Part model, mm, in its own coordinate system. A direction names the side the tool comes from. Coordinates: 2 decimals unless noted, no trailing zeros. Write each loop counter-clockwise with the first axis right and the second up, starting at its lowest first coordinate (ties: lowest second). Pieces come first, ordered by that corner, then holes. Notation, with made-up numbers: (-37.75, -2.75) -> (-1.75, -2.75) arc R34 cw to (-1.75, 31.25) -> close; hole circle Ø6 at (0.25, 1.5). An arc over 180 degrees is marked (long way). Write item = value, one per line.
from build123d import *
from OCP.BRepFilletAPI import BRepFilletAPI_MakeFillet

# Parameters (mm, degrees)
BOSS_EXTRUDE1_DEPTH                                 = 20
CBORE_FOR_M4_HEX_SOCKET_HEAD_CAP_SCREW1_D           = 4.5
CBORE_FOR_M4_HEX_SOCKET_HEAD_CAP_SCREW1_DEPTH       = 10
CBORE_FOR_M4_HEX_SOCKET_HEAD_CAP_SCREW1_CBORE_D     = 8
CBORE_FOR_M4_HEX_SOCKET_HEAD_CAP_SCREW1_CBORE_DEPTH = 4.4
BOSS_EXTRUDE3_DEPTH                                 = 7.8
CUT_EXTRUDE1_DEPTH                                  = 2.4
FILLET3_R                                           = 0.5
CUT_SWEEP1_START                                    = -2.5
CUT_SWEEP1_DEPTH                                    = 5
CUT_EXTRUDE2_REACH                                  = 67.401
SKETCH14_R                                          = 4
FILLET4_R1                                          = 1
FILLET4_R2                                          = 5


# Read off the part's stored shape, not the designer's step: Cut-Sweep1
with BuildPart() as part:
    # Sketch1 → Boss-Extrude1 (new, symmetric)
    with BuildSketch(Plane.XY):
        Polygon((-12.5, 10), (7.5, 10), (7.5, 50), (-7.5, 50), (-7.5, 53), (12.5, 53), (12.5, 0), (-12.5, 0), align=None)
    extrude(amount=BOSS_EXTRUDE1_DEPTH, both=True)

    # CBORE for M4 Hex Socket Head Cap Screw1
    with Locations(Plane(origin=(0, 10, 0), x_dir=(1, 0, 0), z_dir=(0, 1, 0))):
        with Locations((0, -13)):
            CounterBoreHole(CBORE_FOR_M4_HEX_SOCKET_HEAD_CAP_SCREW1_D / 2, CBORE_FOR_M4_HEX_SOCKET_HEAD_CAP_SCREW1_CBORE_D / 2, CBORE_FOR_M4_HEX_SOCKET_HEAD_CAP_SCREW1_CBORE_DEPTH, depth=CBORE_FOR_M4_HEX_SOCKET_HEAD_CAP_SCREW1_DEPTH)

    # Sketch5 → Boss-Extrude3 (add)
    with BuildSketch(Plane(origin=(0, 0, -20), x_dir=(-1, 0, 0), z_dir=(0, 0, -1))):
        Polygon((-5, -8), (5, -8), (8.25, -4.4), (8.25, -2.4), (3.9, -2.4), (3.9, 0), (-3.9, 0), (-3.9, -2.4), (-8.25, -2.4), (-8.25, -4.4), align=None)
    extrude(amount=-BOSS_EXTRUDE3_DEPTH)

    # Sketch6 → Cut-Extrude1 (cut)
    with BuildSketch(Plane(origin=(0, -2.4, 0), x_dir=(1, 0, 0), z_dir=(0, 1, 0))):
        with BuildLine():
            ThreePointArc((-3.9, 16.1), (-2.757716447, 18.857716447), (0, 20))
            Line((0, 20), (-3.9, 20))
            Line((-3.9, 20), (-3.9, 16.1))
        make_face()
        with BuildLine():
            Line((3.9, 12.2), (3.9, 16.1))
            ThreePointArc((3.9, 16.1), (2.757716447, 13.342283553), (0, 12.2))
            Line((0, 12.2), (3.9, 12.2))
        make_face()
    extrude(amount=CUT_EXTRUDE1_DEPTH, mode=Mode.SUBTRACT)

    # Fillet3
    fillet3_edges = [part.edges().sort_by_distance(p)[0] for p in [
        (3.9, 0, -18.05),
        (2.757716447, 0, -13.342283553),
        (-1.95, 0, -12.2),
    ]]
    fillet(fillet3_edges, radius=FILLET3_R)
    fillet3_2_edges = [part.edges().sort_by_distance(p)[0] for p in [
        (-3.9, 0, -14.15),
        (-2.757716447, 0, -18.857716447),
    ]]
    fillet(fillet3_2_edges, radius=FILLET3_R)
    fillet3_3_edges = [part.edges().sort_by_distance(p)[0] for p in [
        (-8.25, -2.4, -16.1),
    ]]
    fillet(fillet3_3_edges, radius=FILLET3_R)
    fillet3_4_edges = [part.edges().sort_by_distance(p)[0] for p in [
        (-8.25, -4.4, -16.1),
    ]]
    fillet(fillet3_4_edges, radius=FILLET3_R)
    fillet3_5_edges = [part.edges().sort_by_distance(p)[0] for p in [
        (-5, -8, -16.1),
    ]]
    fillet(fillet3_5_edges, radius=FILLET3_R)
    fillet3_6_edges = [part.edges().sort_by_distance(p)[0] for p in [
        (5, -8, -16.1),
    ]]
    fillet(fillet3_6_edges, radius=FILLET3_R)
    fillet3_7_edges = [part.edges().sort_by_distance(p)[0] for p in [
        (8.25, -4.4, -16.1),
    ]]
    fillet(fillet3_7_edges, radius=FILLET3_R)
    fillet3_8_edges = [part.edges().sort_by_distance(p)[0] for p in [
        (8.25, -2.4, -16.1),
    ]]
    fillet(fillet3_8_edges, radius=FILLET3_R)

    # Cut-Sweep1 outline → Cut-Sweep1 (cut)
    with BuildSketch(Plane.XY.offset(CUT_SWEEP1_START)):
        with BuildLine():
            Line((12.500000017, 40.338970285), (12.5, 45.105483834))
            add(Edge.make_bspline(
                [(12.5, 45.105483834), (12.059714128, 45.789978249), (11.581411154, 46.38791258), (10.025035585, 47.892146935), (8.787180136, 48.5), (7.5, 48.5)],
                knots=[0.656472281, 0.656472281, 0.656472281, 0.656472281, 0.6875, 0.6875, 0.75, 0.75, 0.75, 0.75], degree=3))
            Line((7.5, 48.5), (7.5, 46.5))
            add(Edge.make_bspline(
                [(12.500000017, 40.338970285), (12.309154865, 40.920252732), (12.103143429, 41.469478304), (11.227294674, 43.513125401), (10.449149583, 44.700789342), (8.901182872, 46.196896563), (8.176315005, 46.5), (7.5, 46.5)],
                knots=[0.604163443, 0.604163443, 0.604163443, 0.604163443, 0.625, 0.625, 0.6875, 0.6875, 0.75, 0.75, 0.75, 0.75], degree=3))
        make_face()
        with BuildLine():
            Line((12.5, 14.894516166), (12.500000017, 19.661029715))
            add(Edge.make_bspline(
                [(7.5, 13.5), (8.176315005, 13.5), (8.901182872, 13.803103437), (10.449149583, 15.299210658), (11.227294674, 16.486874599), (12.103143429, 18.530521696), (12.309154865, 19.079747268), (12.500000017, 19.661029715)],
                knots=[0.25, 0.25, 0.25, 0.25, 0.3125, 0.3125, 0.375, 0.375, 0.395836557, 0.395836557, 0.395836557, 0.395836557], degree=3))
            Line((7.5, 13.5), (7.5, 11.5))
            add(Edge.make_bspline(
                [(7.5, 11.5), (8.787180136, 11.5), (10.025035585, 12.107853065), (11.581411154, 13.61208742), (12.059714128, 14.210021751), (12.5, 14.894516166)],
                knots=[0.25, 0.25, 0.25, 0.25, 0.3125, 0.3125, 0.343527719, 0.343527719, 0.343527719, 0.343527719], degree=3))
        make_face()
    extrude(amount=CUT_SWEEP1_DEPTH, mode=Mode.SUBTRACT)

    # Sketch14 → Cut-Extrude2 (cut, up to next)
    with BuildSketch(Plane(origin=(0, 53, 0), x_dir=(1, 0, 0), z_dir=(0, 1, 0)), mode=Mode.PRIVATE) as cut_extrude2_sk1:
        Polygon((-7.5, -20), (5.5, -20), (5.5, -9), (0, -9), (-7.5, -9), align=None)
        with BuildLine():
            ThreePointArc((4, -13), (-2.828427125, -15.828427125), (0, -9))
            ThreePointArc((0, -9), (2.828427125, -10.171572875), (4, -13))
        make_face(mode=Mode.SUBTRACT)
    cut_extrude2_tool1 = extrude(cut_extrude2_sk1.sketch, amount=-CUT_EXTRUDE2_REACH, mode=Mode.PRIVATE) & part.part
    # Sketch14 → Cut-Extrude2 (cut, up to next)
    with BuildSketch(Plane(origin=(0, 53, 0), x_dir=(1, 0, 0), z_dir=(0, 1, 0)), mode=Mode.PRIVATE) as cut_extrude2_sk2:
        with Locations(Location((0, -13, 0), (0, 0, 270))):
            Circle(SKETCH14_R)
    cut_extrude2_tool2 = extrude(cut_extrude2_sk2.sketch, amount=-CUT_EXTRUDE2_REACH, mode=Mode.PRIVATE) & part.part
    add(cut_extrude2_tool1.solids().sort_by_distance((-1, 53, 19.829706))[0], mode=Mode.SUBTRACT)
    add(cut_extrude2_tool2.solids().sort_by_distance((0, 53, 13))[0], mode=Mode.SUBTRACT)

    # Fillet4: one fillet with a radius per group of edges: ONE call of the kernel's fillet builder (fillet() takes one radius for all edges)
    fillet4_edges_1 = [part.edges().sort_by_distance(p)[0] for p in [
        (-12.5, 10, 0),
        (7.5, 10, 0),
        (7.5, 50, 0),
        (12.5, 53, 0),
        (12.5, 0, 0),
        (-12.5, 0, 0),
        (-7.5, 51.5, 9),
        (-7.5, 51.5, -20),
    ]]
    fillet4_edges_2 = [part.edges().sort_by_distance(p)[0] for p in [
        (5.5, 51.5, 9),
    ]]
    fillet4 = BRepFilletAPI_MakeFillet(part.part.solid().wrapped)
    for e in fillet4_edges_1:
        fillet4.Add(FILLET4_R1, e.wrapped)
    for e in fillet4_edges_2:
        fillet4.Add(FILLET4_R2, e.wrapped)
    add(Compound.cast(fillet4.Shape()), mode=Mode.REPLACE)


solid = part.part
Q1. Saw through at B-B on z = 13. Give the cut face in (x, y), and give its area (3 significant figures).
Model answer:
outline = (-12.5, 1) arc R1 ccw to (-11.5, 0) -> (-2.25, 0) -> (-2.25, 5.6) -> (-4, 5.6) -> (-4, 10) -> (-11.5, 10) arc R1 ccw to (-12.5, 9) -> close; (2.25, 0) -> (11.5, 0) arc R1 ccw to (12.5, 1) -> (12.5, 52) arc R1 ccw to (11.5, 53) -> (5.4, 53) -> (5.4, 50) -> (6.5, 50) arc R1 cw to (7.5, 49) -> (7.5, 11) arc R1 cw to (6.5, 10) -> (4, 10) -> (4, 5.6) -> (2.25, 5.6) -> close
area = 410 mm²
Q2. Probe line 1 (Z direction, x = 0, y = 3.95); line 2 (X direction, y = 2.3, z = 13); line 3 (Y direction, x = 8.25, z = 0). List the from-to ranges inside material, lowest first. Write a range as from..to.
Model answer:
line_1 = -20..10.75, 15.25..20
line_2 = -12.5..-2.25, 2.25..12.5
line_3 = 0..11.57, 13.62..46.38, 48.43..53
Q3. Pin check, flat tips, straight feed: pin 1 (11.5 mm diameter, centred on x = -1.5, z = 0, fed in from -Y); pin 2 (19 mm diameter, centred on y = 21, z = -3.5, fed in from -X); pin 3 (3.5 mm diameter, centred on x = -4, y = 51.5, fed in from +Z). Stop position of each tip, or through.
Model answer:
pin_1 = 0
pin_2 = 7.5
pin_3 = 9
Q4. Mould opens along X. For faces 5 (the face through (0, 50, -4)), 6 (the face through (10, 46, -2.5)), 7 (the face through (10, 46, 2.5)), 8 (the face through (-8.25, -4, -16)) say: released by +X, released by -X, zero draft, split by the parting line, or undercut.
Model answer:
face_5 = zero draft
face_6 = undercut
face_7 = undercut
face_8 = released by -X
Q5. Saw through at D-D on x = -9.25. Give the cut face in (y, z).
Model answer:
outline = (0, -20) -> (10, -20) -> (10, 20) -> (0, 20) -> close
Q6. Saw through at A-A on y = 6.5. Give the cut face in (x, z).
Model answer:
outline = (-12.5, -20) -> (12.5, -20) -> (12.5, 20) -> (-12.5, 20) -> close; hole circle Ø8 at (0, 13)
Q7. Which spindle directions (+Z, -Z, +X, -X, +Y, -Y) get a long thin tool onto all of the face, cutting with end or side? Do faces 1 (the face through (-0.867, 7.831, 16.905)), 2 (the face through (-3, 52, 9)), 3 (the face through (-3.9, -1, -14)), 4 (the face through (-7.5, 51, -5)). Say none if no direction does.
Model answer:
face_1 = +Y
face_2 = +Z, -X, +Y
face_3 = +Z, -Z, -X
face_4 = +Z, -Z, -X, +Y
Q8. Saw through at C-C on y = 29. Give the cut face in (x, z).
Model answer:
outline = (7.5, -20) -> (12.5, -20) -> (12.5, 20) -> (7.5, 20) -> close
